Build history of the part. All positions in model axes, mm. A direction names the side the tool comes from. Round coordinates to 2 decimals unless told otherwise and drop trailing zeros. Write each loop counter-clockwise with the first axis right and the second up, starting at its lowest first coordinate (ties: lowest second). Pieces come first, ordered by that corner, then holes. Notation, with made-up numbers: M 6.5,-10 L 43.5,-10 A25 cw 43.5,8 Z; hole C 64,37 d3. An arc over 180 degrees is marked long. Write item = value, one per line. Start each with the question number.
Q1. Tool access for faces 1 (the flat face through (-11, 23, -2)), 2 (the flat face through (-6, 2, -18.2)), 3 (the flat face through (-5.5, 18.9, -24.5)), 4 (the flat face through (-5, 23, -16)): list every direction of +Z, -Z, +X, -X, +Y, -Y with a clear straight run to the whole face (end or side of a thin tool).
Q2. Pull direction Z, two halves, no side cores. Call faces 5 (the flat face through (-6, 21, -23.2)), 6 (the flat face through (-5, 17.3, -24)), 7 (the cylindrical face through (-5.09, 18.11, -25.11)): released by +Z, released by -Z, zero draft, split by the parting line, or undercut.
Q3. Drop flat-ended pins along their axis: P1, Ø1.2, axis at x = -3, y = 20.5, coming from the -Z side; P2, Ø1.9, axis at x = -9, z = -4, coming from the +Y side; P3, Ø2.5, axis at x = -5.55, z = -26, coming from the +Y side; P4, Ø1, axis at x = -3, z = -17, coming from the -Y side. Give the stop position or say it passes through.
Q4. Probe L1, parallel to Z at x = -5.55, y = 18.2; L2, parallel to X at y = 18.45, z = -26; L3, parallel to Y at x = -1.75, z = -0.5. List the from-to ranges inside material, lowest first.
Q5. Band-saw the part on D-D on y = 6. Write the cut outline in (x, z).
Q6. Band-saw the part on B-B on z = -12.5. Write the cut outline in (x, y).
Q7. Band-saw the part on A-A on z = 2.8. Write the cut outline in (x, y), plus the area to 3 significant figures.
Q8. Band-saw the part on C-C on x = -10.75. Write the cut outline in (y, z), plus the area to 3 significant figures.
Autodesk Inventor part; units mm, degrees
ref_plane "YZ Plane" through (0, 0, 0) normal (1, 0, 0) x (0, 1, 0)
ref_plane "XZ Plane" through (0, 0, 0) normal (0, 1, 0) x (-1, 0, 0)
ref_plane "XY Plane" through (0, 0, 0) normal (0, 0, 1) x (1, 0, 0)
sketch "Boceto1" plane through (0, 0, 0) normal (0, 1, 0) x (-1, 0, 0)
  line L0 (0, 0) -> (11.8, 0)
  line L1 (11.8, 0) -> (11.8, -23.2)
  line L2 (11.8, -23.2) -> (0, -23.2)
  line L3 (0, -23.2) -> (0, 0)
  dimension "d0" = 11.8
  dimension "d1" = 23.2
extrude "Extrusión1" add sketch "Boceto1" along normal blind 23
sketch "Boceto2" plane through (0, 0, 0) normal (1, 0, 0) x (0, 0, -1)
  line L0 (0, 0) -> (0, 23)
  line L1 (0, 0) -> (0, 17.3)
  line L2 (0, 17.3) -> (-4.7, 17.3)
  line L3 (-4.7, 17.3) -> (-4.7, 18.9)
  line L4 (-4.7, 18.9) -> (0, 18.9)
  line L5 (23.2, 0) -> (23.2, 23)
  line L6 (23.2, 17.3) -> (27.9, 17.3)
  line L7 (27.9, 17.3) -> (27.9, 18.9)
  line L8 (27.9, 18.9) -> (23.2, 18.9)
  line L9 (0, 18.9) -> (0, 17.3)
  line L10 (23.2, 18.9) -> (23.2, 17.3)
  line L11 (0, 23) -> (23.2, 23)
  dimension "d4" = 17.3
  dimension "d5" = 4.7
  dimension "d6" = 1.6
  dimension "d7" = 4.7
  dimension "d35" = 4.1
  dimension "d36" = 23
extrude "Extrusión2" add sketch "Boceto2" against normal blind 11.8
move faces "Desplazar1" translate (0.7, 0, 0) faces at (0, 11.5333, -15.4667)
sketch "Boceto4" plane through (-11.8, 18.9, 4.7) normal (0, 1, 0) x (1, 0, 0)
  line L0 (12.5, 0) -> (12.5, 4.7)
  line L1 (0, 0) -> (12.5, 0)
  line L2 (12.5, 0) -> (0, 0)
  line L3 (6.25, 0) -> (6.25, 1.9)
  line L4 (0, 32.6) -> (0, 27.9)
  line L5 (12.5, 32.6) -> (0, 32.6)
  line L6 (0, 32.6) -> (12.5, 32.6)
  line L7 (6.25, 32.6) -> (6.25, 30.7)
  circle A0 centre (6.25, 1.9) radius 1
  circle A1 centre (6.25, 30.7) radius 1
  point P0 (11.8, 4.7)
  dimension "d13" = 1.9
  dimension "d14" = 1.9
  dimension "d15" = 2
  dimension "d16" = 2
extrude "Extrusión3" cut sketch "Boceto4" against normal blind 2.4
sketch "Boceto5" plane through (0, 23, 0) normal (0, 1, 0) x (1, 0, 0)
  line L0 (-11.8, 23.2) -> (-11.8, 0)
  line L1 (-11.8, 0) -> (0.7, 0)
  line L2 (-11.8, 0) -> (0.7, 0)
  line L3 (0.7, 0) -> (0.7, 15)
  line L4 (0.7, 0) -> (0.7, 23.2)
  line L5 (0.7, 15) -> (-11.8, 15)
  line L6 (-11.8, 15) -> (-11.8, 0)
  point P0 (0, 0)
  dimension "d19" = 15
extrude "Extrusión4" add sketch "Boceto5" along normal blind 4
sketch "Boceto6" plane through (0, 27, 0) normal (0, 1, 0) x (1, 0, 0)
  line L0 (-11.8, 0) -> (0.7, 0)
  line L1 (-5.55, 0) -> (-5.55, 5)
  circle A0 centre (-5.55, 5) radius 2.4
  point P0 (0, 0)
  dimension "d22" = 5
  dimension "d23" = 4.8
extrude "Extrusión5" add sketch "Boceto6" along normal blind 3.5
sketch "Boceto7" plane through (0, 27, 0) normal (0, 1, 0) x (1, 0, 0)
  line L0 (-11.8, 0) -> (0.7, 0)
  line L1 (-5.55, 0) -> (-5.55, 6.25)
  arc A0 (-7.9995, 12) -> (-3.1005, 12) centre (-5.55, 6.25) ccw
  line L2 (0.7, 15) -> (-11.8, 15)
  arc A1 (-3.1005, 12) -> (-7.9995, 12) centre (-5.55, 12.5) ccw
  line L3 (0.7, 0) -> (-11.8, 0)
  line L4 (-11.8, 15) -> (-11.8, 0)
  line L5 (-11.8, 0) -> (-11.8, 15)
  line L6 (-11.8, 15) -> (0.7, 15)
  line L7 (0.7, 23.2) -> (0.7, 0)
  line L8 (0.7, 0) -> (0.7, 15)
  point P0 (0, 0)
  dimension "d26" = 6.25
extrude "Extrusión6" cut sketch "Boceto7" against normal up to surface (4 mm away) contours L4 A0 L0 | A0 L7 L0 | L4 L2 A1 A0 | A0 A1 L2 L7
sketch "Boceto8" plane through (-11.8, 0, -23.2) normal (0, 0, -1) x (-1, 0, 0)
  line L0 (-12.5, 0) -> (0, 0)
  line L1 (-12.5, 0) -> (0, 0)
  line L2 (-6.25, 0) -> (-6.25, 3)
  line L3 (-6.25, 3) -> (-8.75, 3)
  line L4 (-8.75, 3) -> (-8.75, 0)
  line L5 (-6.25, 3) -> (-3.75, 3)
  line L6 (-3.75, 3) -> (-3.75, 0)
  point P0 (-11.8, 0)
  dimension "d30" = 3
  dimension "d31" = 2.5
  dimension "d32" = 2.5
extrude "Extrusión7" cut sketch "Boceto8" against normal blind 5
properties part number "microservo_FT"
Conclusion:
q1.face_1 = +Z, -X, +Y
q1.face_2 = -Z, -Y
q1.face_3 = -Z, +X, -X, +Y
q1.face_4 = -Z, +Y
q2.face_5 = released by -Z
q2.face_6 = zero draft
q2.face_7 = undercut
q3.P1 = -23.2
q3.P2 = 27
q3.P3 = 18.9
q3.P4 = 0
q4.L1 = -27.9 to -27, -25 to 1.8, 3.8 to 4.7
q4.L2 = -11.8 to -6.55, -4.55 to 0.7
q4.L3 = 0 to 23
q5.outline = M -11.8,-23.2 L 0.7,-23.2 L 0.7,0 L -11.8,0 Z
q6.outline = M -11.8,0 L 0.7,0 L 0.7,23 L -3.05,23 L -3.05,27 L -8.05,27 L -8.05,23 L -11.8,23 Z
q7.outline = M -11.8,17.3 L -6.55,17.3 L -6.55,18.9 L -11.8,18.9 Z; M -4.55,17.3 L 0.7,17.3 L 0.7,18.9 L -4.55,18.9 Z
q7.area = 16.8 mm^2
q8.outline = M 0,-23.2 L 17.3,-23.2 L 17.3,-27.9 L 18.9,-27.9 L 18.9,-23.2 L 23,-23.2 L 23,-9.72 L 27,-9.72 L 27,-2.78 L 23,-2.78 L 23,0 L 18.9,0 L 18.9,4.7 L 17.3,4.7 L 17.3,0 L 0,0 Z
q8.area = 576 mm^2
